```python
from build123d import *

# Parameters (mm, degrees)
SKETCH_1_W          = 500
SKETCH_1_H          = 140
EXTRUDE_1_DEPTH     = 80
SKETCH_2_W          = 460
SKETCH_2_H          = 100
CUT_EXTRUDE_1_DEPTH = 60
SKETCH_6_R          = 20
SKETCH_6_R_2        = 10
EXTRUDE_4_DEPTH     = 15
CUT_EXTRUDE_2_DEPTH = 517.139516023
SKETCH_8_W          = 460
SKETCH_8_H          = 18.765324385
CUT_EXTRUDE_3_DEPTH = 15


with BuildPart() as part:
    # 草圖1 → 填料-伸長1 (new body)
    with BuildSketch(Plane(origin=(0, 0, 0), x_dir=(1, 0, 0), z_dir=(0, 1, 0))):
        Rectangle(SKETCH_1_W, SKETCH_1_H)
    extrude(amount=EXTRUDE_1_DEPTH)

    # 草圖2 → 除料-伸長1 (cut)
    with BuildSketch(Plane.XZ):
        Rectangle(SKETCH_2_W, SKETCH_2_H)
    extrude(amount=-CUT_EXTRUDE_1_DEPTH, mode=Mode.SUBTRACT)

    # 草圖6 → 伸長-薄件4 (add)
    with BuildSketch(Plane.XZ):
        with Locations((0.114006629, 80)):
            Circle(SKETCH_6_R)
        with Locations((0.114006629, 80)):
            Circle(SKETCH_6_R_2, mode=Mode.SUBTRACT)
    extrude(amount=-EXTRUDE_4_DEPTH)

    # 草圖7 → 除料-伸長2 (cut, through all)
    with BuildSketch(Plane(origin=(250, 0, 0), x_dir=(0, 0, -1), z_dir=(1, 0, 0))):
        Polygon((-70, 21.729405289), (31.457073642, 80), (-70, 80), align=None)
    extrude(amount=-CUT_EXTRUDE_2_DEPTH, mode=Mode.SUBTRACT)

    # 草圖8 → 除料-伸長3 (cut)
    with BuildSketch(Plane(origin=(0, 46.570964705, 26.747448081), x_dir=(1, 0, 0), z_dir=(0, 0.8671544755717103, 0.4980392710378893))):
        with Locations((0, 36.346470221)):
            Rectangle(SKETCH_8_W, SKETCH_8_H)
    extrude(amount=-CUT_EXTRUDE_3_DEPTH, mode=Mode.SUBTRACT)


solid = part.part
```
For this review, take the finished solid that the model builds, in its own axes (mm). A direction names the side the tool comes from. Round coordinates to 2 decimals unless told otherwise and drop trailing zeros. Loops run counter-clockwise (first coordinate to the right, second up) from the corner with the lowest first, then second, coordinate; pieces in that order, holes last.
Q1. Add section C-C on y = 48. Write out the cut boundary in (x, z), plus the area to 3 significant figures.
Result sheet:
outline: (-250, -70) - (250, -70) - (250, 24.26) - (230, 24.26) - (230, -50) - (-230, -50) - (-230, 24.26) - (-250, 24.26) - close
area: 13,000 mm2
Q2. Add section A-A on x = -80.5. Write out the cut boundary in (y, z), plus the area to 3 significant figures.
Result sheet:
outline: (0, -70) - (80, -70) - (80, -31.46) - (69.35, -12.91) - (60, -18.27) - (60, -50) - (0, -50) - close; (0, 50) - (33.22, 50) - (21.73, 70) - (0, 70) - close
area: 2,770 mm2
Q3. Add section D-D on z = 29. Write out the cut boundary in (x, y).
Result sheet:
outline: (-250, 0) - (-230, 0) - (-230, 45.28) - (-250, 45.28) - close; (230, 0) - (250, 0) - (250, 45.28) - (230, 45.28) - close
Q4. Add section B-B on z = 80. Write out the cut boundary in (x, y).
Result sheet:
outline: (-19.89, 0) - (-9.89, 0) - (-9.89, 15) - (-19.89, 15) - close; (10.11, 0) - (20.11, 0) - (20.11, 15) - (10.11, 15) - close
Q5. Machinability: for faces 4 (the face through (-3, 16, 50)), 5 (the face through (-3.22, 64.74, -15.55)), 6 (the face through (0, 15, 92)), 7 (the face through (-230, 26, -1)), which of the approach directions +Z, -Z, +X, -X, +Y, -Y give a long, thin tool a straight path to every point of the face, cutting with its end or side? Answer none if there is none.
Result sheet:
face 4: +Y, -Y
face 5: +Z, -Y
face 6: +Z, +X, -X, +Y
face 7: -Y
Q6. Mouldability with a two-part tool opening along Z and no side actions: class faces 1 (the face through (230, 26, -1)), 2 (the face through (3.5, 31.033, 53.801)), 3 (the face through (-3, 60, -34)) as +Z half, -Z half, draft (parallel to the pull), parting line (faces both ways), or undercut.
Result sheet:
face 1: undercut
face 2: +Z half
face 3: draft
Q7. To check wall thickness, follow line 1 along X through (y, z) = (7, 80); line 2 along X through (y, z) = (23.5, -29); line 3 along Z through (x, y) = (-222, 9.5). State the ranges of each line that lie inside material, in increasing order.
Result sheet:
line 1: x = -19.89 to -9.89, 10.11 to 20.11
line 2: x = -250 to -230, 230 to 250
line 3: z = -70 to -50, 50 to 70
Q8. Insertion check: pin 1 Ø9.5 at (x, z) = (19.5, -40) entering from -Y; pin 2 Ø4 at (x, y) = (-189.5, 63.5) entering from +Z; pin 3 Ø17.5 at (x, y) = (102, 7.5) entering from +Z. Each pin has a flat end and moves straight along its axis. Give the tip position at first contact, or say it passes through.
Result sheet:
pin 1: stops at y = 60
pin 2: stops at z = -15.12
pin 3: stops at z = 70
